Geometry: final body of the model. Coordinates: model frame, mm. A direction names the side the tool comes from. Round coordinates to 2 decimals unless told otherwise and drop trailing zeros. Loops run counter-clockwise (first coordinate to the right, second up) from the corner with the lowest first, then second, coordinate; pieces in that order, holes last. Notation, with made-up numbers: (65, -18) - (96, -18) arc R22 cw to (96, 20) - close; hole circle Ø10 at (45.25, 37.5). An arc over 180 degrees is marked (long way). Answer in a Markdown table with one row per item. Add a question column.
from build123d import *

# Parameters (mm, degrees)
F0_W     = 12.7
F0_H     = 25.4
F1_DEPTH = 25.4
F3_DEPTH = 12.7
F4_W     = 12.7
F4_H     = 12.7
F5_DEPTH = 12.7
F6_R     = 6.35
F6_R_2   = 3.175
F7_DEPTH = 25.4


with BuildPart() as f1:
    # F0 (on Front) → F1 (new body)
    with BuildSketch(Plane.XZ):
        with Locations((6.35, 12.7)):
            Rectangle(F0_W, F0_H)
    extrude(amount=-F1_DEPTH)

    # F2 (on face) → F3 (cut)
    with BuildSketch(Plane.YZ.offset(12.7)):
        Polygon((6.35, 25.4), (0, 25.4), (0, 19.05), align=None)
        Polygon((25.4, 25.4), (19.05, 25.4), (25.4, 19.05), align=None)
    extrude(amount=-F3_DEPTH, mode=Mode.SUBTRACT)

    # F4 (on face) → F5 (join)
    with BuildSketch(Plane.YZ.offset(12.7)):
        with Locations((12.7, 12.7)):
            Rectangle(F4_W, F4_H)
    extrude(amount=F5_DEPTH)

    # F6 (on Front) → F7 (join)
    with BuildSketch(Plane.XZ):
        with Locations((25.4, 12.7)):
            Circle(F6_R)
        with Locations((25.4, 12.7)):
            Circle(F6_R_2, mode=Mode.SUBTRACT)
    extrude(amount=-F7_DEPTH)


solid = f1.part
1) Section A-A, the plane z = 12.7. Return the cut outline in (x, y) (3 decimals).
2) Pull-direction query (Z, two-part tool) for faces 1 (the cylindrical face through (28.43, 12.52, 13.65)), 2 (the flat face through (6, 13, 0)), 3 (the flat face through (19, 13, 19.05)); classes: pulls with the +Z half, pulls with the -Z half, needs draft (parallel to the pull), parting line crosses it, or undercut.
3) Section D-D, the plane y = 9.75. Return the cut outline in (x, z) (3 decimals), and give its area (3 significant figures).
4) Section B-B, the plane y = 23.5. Return the cut outline in (x, z) (3 decimals).
5) Reachability of faces 4 (the flat face through (19, 13, 6.35)), 5 (the flat face through (25.4, 13, 13)), 6 (the flat face through (6, 25.4, 10)), 7 (the flat face through (24, 6.35, 13)), 8 (the cylindrical face through (31.457, 12.522, 14.607)) from +Z, -Z, +X, -X, +Y, -Y: full face, straight path, thin tool, end or side. Return the list, or none.
6) Material intervals for line 1 along X through (y, z) = (9.75, 12.7) (3 decimals); line 2 along X through (y, z) = (2.5, 14.5); line 3 along Y through (x, z) = (15, 15.25), sorted ascending. Write a range as from..to.
7) Section C-C, the plane x = 27. Return the cut outline in (y, z), and give its area (3 significant figures).
8) Contact query for flat-ended pins moving along their axis: pin 1 Ø2.5 at (x, z) = (24.5, 13.5) entering from +Y; pin 2 Ø2 at (y, z) = (3.5, 3) entering from +X; pin 3 Ø2 at (x, z) = (14.5, 11) entering from -Y. Output: stop coordinate, or through.
Evaluation:
| question | item | result |
|---|---|---|
| 1 | outline | (0, 0) - (12.7, 0) - (12.7, 6.35) - (19.05, 6.35) - (19.05, 0) - (22.225, 0) - (22.225, 6.35) - (25.4, 6.35) - (25.4, 19.05) - (22.225, 19.05) - (22.225, 25.4) - (19.05, 25.4) - (19.05, 19.05) - (12.7, 19.05) - (12.7, 25.4) - (0, 25.4) - close; (28.575, 0) - (31.75, 0) - (31.75, 25.4) - (28.575, 25.4) - close |
| 2 | face 1 | undercut |
| 2 | face 2 | pulls with the -Z half |
| 2 | face 3 | pulls with the +Z half |
| 3 | outline | (0, 0) - (12.7, 0) - (12.7, 6.35) - (25.4, 6.35) arc R6.35 ccw to (25.4, 19.05) - (12.7, 19.05) - (12.7, 25.4) - (0, 25.4) - close; hole (25.4, 9.525) arc R3.175 ccw to (25.4, 15.875) - close |
| 3 | area | 531 mm² |
| 4 | outline | (0, 0) - (12.7, 0) - (12.7, 20.95) - (0, 20.95) - close; circle Ø12.7 at (25.4, 12.7); hole circle Ø6.35 at (25.4, 12.7) |
| 5 | face 4 | -Z, +X, +Y, -Y |
| 5 | face 5 | +Y, -Y |
| 5 | face 6 | +Z, -Z, +X, -X, +Y |
| 5 | face 7 | -Y |
| 5 | face 8 | none |
| 6 | line 1 | x = 0..25.4, 28.575..31.75 |
| 6 | line 2 | x = 0..12.7, 19.31..22.78, 28.02..31.49 |
| 6 | line 3 | y = 6.35..19.05 |
| 7 | outline | (0, 6.55) - (25.4, 6.55) - (25.4, 9.96) - (0, 9.96) - close; (0, 15.44) - (25.4, 15.44) - (25.4, 18.85) - (0, 18.85) - close |
| 7 | area | 173 mm² |
| 8 | pin 1 | stops at y = 19.05 |
| 8 | pin 2 | stops at x = 12.7 |
| 8 | pin 3 | stops at y = 6.35 |
